Verification items for the finished model (mm, model axes). Face numbers are marked on the shaded views. A direction names the side the tool comes from. Round coordinates to 2 decimals unless told otherwise and drop trailing zeros. Write each loop counter-clockwise with the first axis right and the second up, starting at its lowest first coordinate (ties: lowest second). Pieces come first, ordered by that corner, then holes. Notation, with made-up numbers: M -21.75,71.5 L 30.25,71.5 A22 cw 30.25,83.5 Z; hole C -27,88.25 d6. An arc over 180 degrees is marked long. Answer in a Markdown table with one row per item. Add a question column.
1. Sectioned sample at A-A on x = 19.5. Record the cut outline in (y, z).
2. Sectioned sample at B-B on y = 1.1. Count the separate pieces of the cut face and the enclosed holes in it, plus the area to 3 significant figures.
3. Material ranges on probe 1 along Y at (x, z) = (-8.5, -5.7); probe 2 along X at (y, z) = (-4, -17.5); probe 3 along X at (y, z) = (0, -6.05), recorded low to high.
4. Set-up check for the marked faces 4, 5 and 6: record each of +Z, -Z, +X, -X, +Y, -Y from which the full face is reachable in a straight line by a thin tool's end or side.
5. Sectioned sample at C-C on y = 4.5. Record the cut outline in (x, z), plus the area to 3 significant figures.
6. Draft check along Z on the marked faces 1, 2 and 3. Enter one of: pulls with the +Z half, pulls with the -Z half, needs draft (parallel to the pull), parting line crosses it, or undercut.
7. Go/stop test with flat-tipped pins: pin 1 Ø4 at (x, y) = (12.5, 3.5) entering from +Z; pin 2 Ø6 at (y, z) = (-2, -12) entering from -X; pin 3 Ø3.5 at (x, y) = (20, -1.5) entering from +Z. Record where each tip stops, or that it passes through.
8. Sectioned sample at D-D on z = -18. Record the cut outline in (x, y).
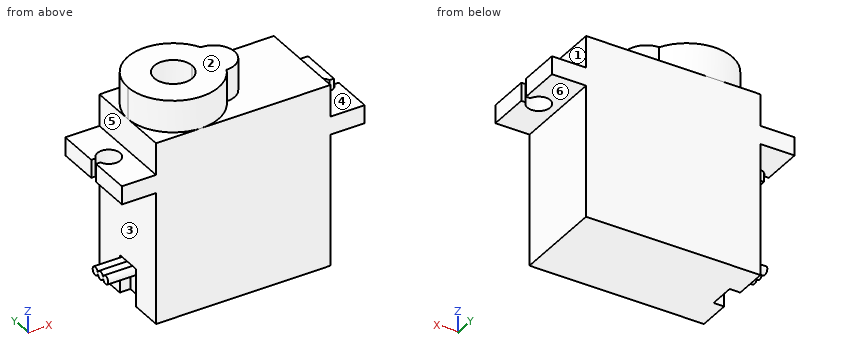
```python
from build123d import *

# Parameters (mm, degrees)
PAD023_DEPTH         = 6
POCKET021_DEPTH      = 62.4829974073
POCKET021_DEPTH_BACK = 86.4829974073
PAD001_DEPTH         = 4.2
SKETCH003_W          = 5
SKETCH003_H          = 3.4
POCKET022_DEPTH      = 1.4
SKETCH004_R          = 0.55
PAD002_DEPTH         = 5


with BuildPart() as part:
    # Sketch044 → Pad023 (new body, symmetric)
    with BuildSketch(Plane.XZ):
        Polygon((-11.5, 0), (0, 0), (0, 24), (-11.5, 24), (-11.5, 19.8), (-16, 19.8), (-16, 17.4), (-11.5, 17.4), align=None)
    extrude(amount=PAD023_DEPTH, both=True)

    # Sketch001 → Pocket021 (cut, two sides)
    with BuildSketch(Plane.XY) as pocket021_sk:
        with BuildLine():
            ThreePointArc((-15.4142135624, -0.5), (-12.5, 0), (-15.4142135624, 0.5))
            Line((-15.4142135624, 0.5), (-19.4142135624, 0.5))
            Line((-19.4142135624, 0.5), (-19.4142135624, -0.5))
            Line((-19.4142135624, -0.5), (-15.4142135624, -0.5))
        make_face()
    extrude(amount=-POCKET021_DEPTH, mode=Mode.SUBTRACT)
    extrude(pocket021_sk.sketch, amount=POCKET021_DEPTH_BACK, mode=Mode.SUBTRACT)

    # Mirrored007: part across Sketch001 V_Axis


with BuildPart() as part_1:
    add(part.part)
    add(part.part.mirror(Plane(origin=(0, 0, 0), x_dir=(0, 0, 1), z_dir=(1, 0, 0))))

    # Sketch002 (on Face22 of Mirrored007) → Pad001 (join)
    with BuildSketch(Plane(origin=(-5.5, 0, 24), x_dir=(-1, 0, 0), z_dir=(0, 0, 1))):
        with BuildLine():
            ThreePointArc((6, 0), (1.41490397, 5.8307844031), (-5.3326822519, 2.75))
            ThreePointArc((-5.3326822519, 2.75), (-7.2772259002, 1.9445436483), (-8.0826822519, 0))
            Line((-8.0826822519, 0), (-2.5, 0))
            ThreePointArc((2.5, 0), (0, 2.5), (-2.5, 0))
            Line((2.5, 0), (6, 0))
        make_face()
    pad001 = extrude(amount=PAD001_DEPTH)

    # Mirrored008: Pad001 across Sketch002 H_Axis
    add(pad001.mirror(Plane(origin=(-5.5, 0, 24), x_dir=(0, 0, 1), z_dir=(0, -1, 0))))

    # Sketch003 (on Face3 of Mirrored008) → Pocket022 (cut)
    with BuildSketch(Plane(origin=(-11.5, 0, 0), x_dir=(0, 0, -1), z_dir=(-1, 0, 0))):
        with Locations((-2.5, 0)):
            Rectangle(SKETCH003_W, SKETCH003_H)
    extrude(amount=-POCKET022_DEPTH, mode=Mode.SUBTRACT)

    # Sketch004 (on Face28 of Pocket022) → Pad002 (join)
    with BuildSketch(Plane(origin=(-10.1, 0, 0), x_dir=(0, 0, -1), z_dir=(-1, 0, 0))):
        with Locations((-4.4, 1.1)):
            Circle(SKETCH004_R)
        with Locations((-4.4, 0)):
            Circle(SKETCH004_R)
        with Locations((-4.4, -1.1)):
            Circle(SKETCH004_R)
    extrude(amount=PAD002_DEPTH)


with BuildPart() as part_2:
    # Body018 placement: moved
    add(part_1.part.moved(Location((5.5, 0, -24))))


solid = part_2.part
```
Geometry check:
| question | item | result |
|---|---|---|
| 1 | outline | M -6,-6.6 L -1.5,-6.6 L -1.5,-4.2 L -6,-4.2 Z; M 1.5,-6.6 L 6,-6.6 L 6,-4.2 L 1.5,-4.2 Z |
| 2 | separate pieces | 3 |
| 2 | enclosed holes | 0 |
| 2 | area | 601 mm2 |
| 3 | probe 1 | y = -6 to -1.5, 1.5 to 6 |
| 3 | probe 2 | x = -6 to 17 |
| 3 | probe 3 | x = -7 to 18 |
| 4 | face 4 | +Z, +X, +Y, -Y |
| 4 | face 5 | +Z, -X, +Y, -Y |
| 4 | face 6 | -Z, +X, +Y, -Y |
| 5 | outline | M -10.5,-6.6 L -6,-6.6 L -6,-24 L 17,-24 L 17,-6.6 L 21.5,-6.6 L 21.5,-4.2 L 17,-4.2 L 17,0 L 3.97,0 L 3.97,4.2 L -3.97,4.2 L -3.97,0 L -6,0 L -6,-4.2 L -10.5,-4.2 Z |
| 5 | area | 607 mm2 |
| 6 | face 1 | needs draft |
| 6 | face 2 | pulls with the +Z half |
| 6 | face 3 | undercut |
| 7 | pin 1 | stops at z = 0 |
| 7 | pin 2 | stops at x = -6 |
| 7 | pin 3 | stops at z = -4.2 |
| 8 | outline | M -6,-6 L 17,-6 L 17,6 L -6,6 Z |
